The listing builds one solid part. Answer for the finished solid, in the listing's coordinates (mm). Round coordinates to 2 decimals unless told otherwise and drop trailing zeros. Order: outer loops, then holes, each group sorted by start corner. A loop starts at its lowest first (then second) coordinate and runs counter-clockwise, first axis right, second up. Notation, with made-up numbers: (-10.5, 37) - (22.5, 37) arc R9 cw to (22.5, 54) - close; hole circle Ø6 at (7, 60). An arc over 180 degrees is marked (long way). Use CSV: the item, a comma, the result in double quotes. Start each with the question number.
Item 1: Find section A-A, the plane z = 2.2. Give the vertices of the cut face in (x, y).
Item 2: Flat-ended cylindrical pins translate along their axes: P1, Ø2.5, axis at x = -37.95, y = 5.21, coming from the -Z side; P2, Ø3, axis at x = -20.5, y = -11.5, coming from the -Z side; P3, Ø0.5, axis at x = -17, z = -0.5, coming from the +Y side; P4, Ø0.8, axis at y = -5, z = -0.5, coming from the -X side. Find the tip coordinate at first contact, or state that the pin passes through.
Item 3: Find section B-B, the plane x = 0. Give the vertices of the cut face in (y, z).
Item 4: Straight lines are drawn through the part: line 1 along X through (y, z) = (-27, 2.55); line 2 along Y through (x, z) = (-37, 2.25); line 3 along X through (y, z) = (-11.5, 2.45). For each, find the intervals that lie inside material, in ascending order. Write a range as [from, to].
Item 5: Find section C-C, the plane y = -19. Give the vertices of the cut face in (x, z), plus the area to 3 significant figures.
```python
from build123d import *

# Parameters (mm, degrees)
F0_W      = 89
F0_H      = 44
F0_W_2    = 85
F0_H_2    = 40
F1_DEPTH  = 3
F2_R      = 5
F3_W      = 83
F3_H      = 38
F4_DEPTH  = 1
F5_R      = 2
F6_R      = 1.5
F7_DEPTH  = 25
F8_R      = 2.75
F9_DEPTH  = 2.5
F10_R     = 1.5
F11_DEPTH = 25


with BuildPart() as f1:
    # F0 (on Top) → F1 (new body)
    with BuildSketch(Plane.XY):
        with Locations((0.5476979613, -10.7853626366)):
            Rectangle(F0_W, F0_H)
        with Locations((0.5476979613, -10.7853626366)):
            Rectangle(F0_W_2, F0_H_2, mode=Mode.SUBTRACT)
        with Locations((0.5476979613, -10.7853626366)):
            Rectangle(F0_W_2, F0_H_2)
    extrude(amount=F1_DEPTH)

    # F2
    f2_edges = [f1.edges().sort_by_distance(p)[0] for p in [
        (-43.952302, 11.214637, 1.5),
        (45.047698, 11.214637, 1.5),
        (45.047698, -32.785363, 1.5),
        (-43.952302, -32.785363, 1.5),
    ]]
    fillet(f2_edges, radius=F2_R)

    # F3 (on face) → F4 (join)
    with BuildSketch(Plane(origin=(0, 0, 0), x_dir=(1, 0, 0), z_dir=(0, 0, -1))):
        with Locations((0.5476979613, 10.7853626366)):
            Rectangle(F3_W, F3_H)
    extrude(amount=F4_DEPTH)

    # F5
    f5_edges = [f1.edges().sort_by_distance(p)[0] for p in [
        (-40.952302, -29.785363, -0.5),
        (-40.952302, 8.214637, -0.5),
        (42.047698, 8.214637, -0.5),
        (42.047698, -29.785363, -0.5),
    ]]
    fillet(f5_edges, radius=F5_R)

    # F6 (on face) → F7 (cut)
    with BuildSketch(Plane(origin=(0, 0, -1), x_dir=(1, 0, 0), z_dir=(0, 0, -1))):
        with Locations((22.0476979613, 10.7853626366)):
            Circle(F6_R)
        with BuildLine():
            ThreePointArc((-22.4523020387, 10.7853626366), (-20.9523020387, 9.2853626366), (-19.4523020387, 10.7853626366))
            ThreePointArc((-19.4523020387, 10.7853626366), (-20.9523020387, 12.2853626366), (-22.4523020387, 10.7853626366))
        make_face()
    extrude(amount=-F7_DEPTH, mode=Mode.SUBTRACT)

    # F8 (on face) → F9 (cut)
    with BuildSketch(Plane(origin=(0, 0, -1), x_dir=(1, 0, 0), z_dir=(0, 0, -1))):
        with Locations((-20.9523020387, 10.7853626366)):
            Circle(F8_R)
        with Locations((22.0476979613, 10.7853626366)):
            Circle(F8_R)
    extrude(amount=-F9_DEPTH, mode=Mode.SUBTRACT)

    # F10 (on face) → F11 (cut)
    with BuildSketch(Plane.XY.offset(3)):
        with BuildLine():
            ThreePointArc((-36.4523020387, -26.7853626366), (-37.9523020387, -25.2853626366), (-39.4523020387, -26.7853626366))
            Line((-39.4523020387, -26.7853626366), (-37.9523020387, -26.7853626366))
            Line((-37.9523020387, -26.7853626366), (-37.9523020387, -28.2853626366))
            ThreePointArc((-37.9523020387, -28.2853626366), (-36.8916418669, -27.8460228084), (-36.4523020387, -26.7853626366))
        make_face()
        with BuildLine():
            Line((-37.9523020387, -26.7853626366), (-39.4523020387, -26.7853626366))
            ThreePointArc((-39.4523020387, -26.7853626366), (-39.0129622104, -27.8460228084), (-37.9523020387, -28.2853626366))
            Line((-37.9523020387, -28.2853626366), (-37.9523020387, -26.7853626366))
        make_face()
        with Locations((-37.9523020387, 5.2146373634)):
            Circle(F10_R)
        with Locations((39.0476979613, -26.7853626366)):
            Circle(F10_R)
        with Locations((39.0476979613, 5.2146373634)):
            Circle(F10_R)
    extrude(amount=-F11_DEPTH, mode=Mode.SUBTRACT)


solid = f1.part
```
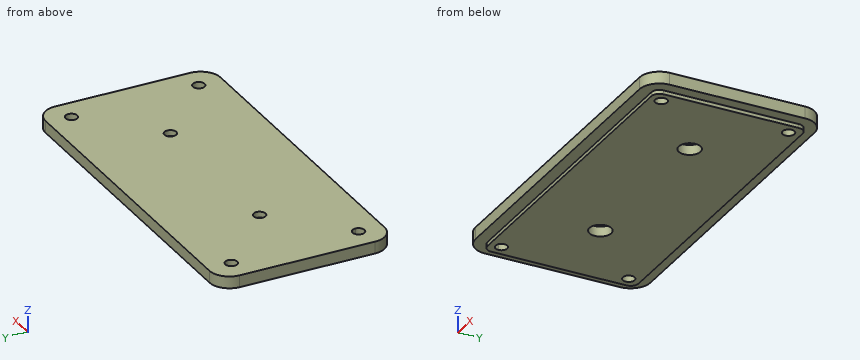
Worked out:
1,outline,"(-43.95, -27.79) arc R5 ccw to (-38.95, -32.79) - (40.05, -32.79) arc R5 ccw to (45.05, -27.79) - (45.05, 6.21) arc R5 ccw to (40.05, 11.21) - (-38.95, 11.21) arc R5 ccw to (-43.95, 6.21) - close; hole circle Ø3 at (-37.95, -26.79); hole circle Ø3 at (-37.95, 5.21); hole circle Ø3 at (-20.95, -10.79); hole circle Ø3 at (22.05, -10.79); hole circle Ø3 at (39.05, -26.79); hole circle Ø3 at (39.05, 5.21)"
2,P1,"passes through"
2,P2,"stops at z = 1.5"
2,P3,"stops at y = 8.21"
2,P4,"stops at x = -40.95"
3,outline,"(-32.79, 0) - (-29.79, 0) - (-29.79, -1) - (8.21, -1) - (8.21, 0) - (11.21, 0) - (11.21, 3) - (-32.79, 3) - close"
4,line 1,"x = [-43.95, -39.44], [-36.47, 37.56], [40.53, 45.05]"
4,line 2,"y = [-32.79, -27.94], [-25.63, 4.06], [6.37, 11.21]"
4,line 3,"x = [-43.95, -22.27], [-19.63, 20.73], [23.37, 45.05]"
5,outline,"(-43.95, 0) - (-40.95, 0) - (-40.95, -1) - (42.05, -1) - (42.05, 0) - (45.05, 0) - (45.05, 3) - (-43.95, 3) - close"
5,area,"350 mm²"
